Geometry: final body of the model. Coordinates: model frame, mm. A direction names the side the tool comes from. Give positions to 0.01 mm unless a question says otherwise; leave off trailing zeros. Write each loop counter-clockwise with the first axis right and the second up, starting at its lowest first coordinate (ties: lowest second). Pieces come first, ordered by that corner, then holes. Notation, with made-up numbers: M 67,-33 L 99,-33 A16 ccw 99,-15 Z; hole C 89,32 d2. An arc over 180 degrees is marked long. Answer as a JSON object with one key per item and string values.
from build123d import *

# Parameters (mm, degrees)
F0_R     = 5
F0_R_2   = 2.5
F0_W     = 28
F0_H     = 8
F1_DEPTH = 10
F2_DEPTH = 3


with BuildPart() as f1:
    # F0 (on Front) → F1 (new body)
    with BuildSketch(Plane.XZ):
        with BuildLine():
            Line((-14, 20), (-26, 20))
            ThreePointArc((-26, 20), (-31.656854, 17.656854), (-34, 12))
            Line((-34, 12), (-34, -12))
            ThreePointArc((-34, -12), (-31.656854, -17.656854), (-26, -20))
            Line((-26, -20), (-14, -20))
            Line((-14, -20), (-14, -12))
            Line((-14, -12), (14, -12))
            Line((14, -12), (14, -20))
            Line((14, -20), (26, -20))
            ThreePointArc((26, -20), (31.656854, -17.656854), (34, -12))
            Line((34, -12), (34, 12))
            ThreePointArc((34, 12), (31.656854, 17.656854), (26, 20))
            Line((26, 20), (14, 20))
            Line((14, 20), (14, 12))
            Line((14, 12), (-14, 12))
            Line((-14, 12), (-14, 20))
        make_face()
        with Locations((-26, -12)):
            Circle(F0_R, mode=Mode.SUBTRACT)
        with Locations((26, -12)):
            Circle(F0_R, mode=Mode.SUBTRACT)
        with Locations((-26, 12)):
            Circle(F0_R, mode=Mode.SUBTRACT)
        with Locations((26, 12)):
            Circle(F0_R, mode=Mode.SUBTRACT)
        with Locations((-26, 12)):
            Circle(F0_R)
        with Locations((-26, 12)):
            Circle(F0_R_2, mode=Mode.SUBTRACT)
        with Locations((26, 12)):
            Circle(F0_R)
        with Locations((26, 12)):
            Circle(F0_R_2, mode=Mode.SUBTRACT)
        with Locations((26, -12)):
            Circle(F0_R)
        with Locations((26, -12)):
            Circle(F0_R_2, mode=Mode.SUBTRACT)
        with Locations((-26, -12)):
            Circle(F0_R)
        with Locations((-26, -12)):
            Circle(F0_R_2, mode=Mode.SUBTRACT)
        with Locations((0, -16)):
            Rectangle(F0_W, F0_H)
        with Locations((0, 16)):
            Rectangle(F0_W, F0_H)
    extrude(amount=-F1_DEPTH)

    # F0 (on Front) → F2 (cut)
    with BuildSketch(Plane.XZ):
        with Locations((-26, 12)):
            Circle(F0_R)
        with Locations((-26, 12)):
            Circle(F0_R_2, mode=Mode.SUBTRACT)
        with Locations((26, 12)):
            Circle(F0_R)
        with Locations((26, 12)):
            Circle(F0_R_2, mode=Mode.SUBTRACT)
        with Locations((26, -12)):
            Circle(F0_R)
        with Locations((26, -12)):
            Circle(F0_R_2, mode=Mode.SUBTRACT)
        with Locations((-26, -12)):
            Circle(F0_R)
        with Locations((-26, -12)):
            Circle(F0_R_2, mode=Mode.SUBTRACT)
    extrude(amount=-F2_DEPTH, mode=Mode.SUBTRACT)


solid = f1.part
1) Cut plane C-C on y = 0.75. Return loops of the section in (x, z), and give its area (3 significant figures).
Geometry check:
{"outline": "M -34,-12 A8 ccw -26,-20 L 26,-20 A8 ccw 34,-12 L 34,12 A8 ccw 26,20 L -26,20 A8 ccw -34,12 Z; hole C -26,-12 d10; hole C -26,12 d10; hole C 26,-12 d10; hole C 26,12 d10", "area": "2,350 mm2"}
2) Pull-direction query (Z, two-part tool) for faces 3 (the cylindrical face through (-31.719, 4.93, -17.594)), 4 (the cylindrical face through (-31.594, 4.93, 17.719)), 5 (the flat face through (28, 3, 10)); classes: pulls with the +Z half, pulls with the -Z half, needs draft (parallel to the pull), parting line crosses it, or undercut.
Geometry check:
{"face 3": "pulls with the -Z half", "face 4": "pulls with the +Z half", "face 5": "undercut"}
3) Set-up query: faces 1 (the cylindrical face through (25.46, 6.45, 9.56)), 2 (the flat face through (-24, 3, -14)). Return all of +Z, -Z, +X, -X, +Y, -Y with unobstructed straight access to the full face (end or side cutting, diameter ignored); none if empty.
Geometry check:
{"face 1": "+Y, -Y", "face 2": "-Y"}
4) Line query: line 1 (Z direction, x = -26, y = 0.8); line 2 (Z direction, x = 26, y = 7); line 3 (Z direction, x = 30.5, y = 3.25). Output: solid intervals per line, ascending. Write a range as from..to.
Geometry check:
{"line 1": "z = -20..-17, -7..7, 17..20", "line 2": "z = -20..-14.5, -9.5..9.5, 14.5..20", "line 3": "z = -18.61..18.61"}
5) Contact query for flat-ended pins moving along their axis: P1, Ø4.5, axis at x = -26, z = 12, coming from the -Y side; P2, Ø3, axis at x = 26, z = 13.5, coming from the -Y side. Output: stop coordinate, or through.
Geometry check:
{"P1": "passes through", "P2": "stops at y = 3"}
6) Cut plane B-B on x = -24.5. Return loops of the section in (y, z), and give its area (3 significant figures).
Geometry check:
{"outline": "M 0,-20 L 10,-20 L 10,-14 L 3,-14 L 3,-16.77 L 0,-16.77 Z; M 0,-7.23 L 3,-7.23 L 3,-10 L 10,-10 L 10,10 L 3,10 L 3,7.23 L 0,7.23 Z; M 0,16.77 L 3,16.77 L 3,14 L 10,14 L 10,20 L 0,20 Z", "area": "287 mm2"}
7) Cut plane A-A on y = 8.75. Return loops of the section in (x, z), and give its area (3 significant figures).
Geometry check:
{"outline": "M -34,-12 A8 ccw -26,-20 L 26,-20 A8 ccw 34,-12 L 34,12 A8 ccw 26,20 L -26,20 A8 ccw -34,12 Z; hole C -26,-12 d5; hole C -26,12 d5; hole C 26,-12 d5; hole C 26,12 d5", "area": "2,590 mm2"}
